from build123d import *

# Parameters (mm, degrees)
SKETCH1_W           = 29.083
SKETCH1_H           = 13.0302
BOSS_EXTRUDE1_DEPTH = 19.0754
SKETCH2_W           = 39.9542
SKETCH2_H           = 13.0302
BOSS_EXTRUDE2_DEPTH = 3.4798
SKETCH3_W           = 29.21
SKETCH3_H           = 12.954
BOSS_EXTRUDE3_DEPTH = 4.0132
SKETCH4_R           = 3.071074645
BOSS_EXTRUDE4_DEPTH = 4.572
SKETCH5_R           = 2.159
CUT_EXTRUDE1_DEPTH  = 3.4798


with BuildPart() as part:
    # Sketch1 → Boss-Extrude1 (new body)
    with BuildSketch(Plane(origin=(0, 0, 0), x_dir=(1, 0, 0), z_dir=(0, 1, 0))):
        Rectangle(SKETCH1_W, SKETCH1_H)
    extrude(amount=BOSS_EXTRUDE1_DEPTH)

    # Sketch2 → Boss-Extrude2 (add)
    with BuildSketch(Plane(origin=(0, 19.0754, 0), x_dir=(1, 0, 0), z_dir=(0, 1, 0))):
        Rectangle(SKETCH2_W, SKETCH2_H)
    extrude(amount=BOSS_EXTRUDE2_DEPTH)

    # Sketch3 → Boss-Extrude3 (add)
    with BuildSketch(Plane(origin=(0, 22.5552, 0), x_dir=(1, 0, 0), z_dir=(0, 1, 0))):
        with Locations((-0.0635, 0.0381)):
            Rectangle(SKETCH3_W, SKETCH3_H)
    extrude(amount=BOSS_EXTRUDE3_DEPTH)

    # Sketch4 → Boss-Extrude4 (add)
    with BuildSketch(Plane(origin=(0, 26.5684, 0), x_dir=(1, 0, 0), z_dir=(0, 1, 0))):
        with Locations(Location((-9.4771, 0, 0), (0, 0, 90))):
            Circle(SKETCH4_R)
    extrude(amount=BOSS_EXTRUDE4_DEPTH)

    # Sketch5 → Cut-Extrude1 (cut)
    with BuildSketch(Plane(origin=(0, 22.5552, 0), x_dir=(1, 0, 0), z_dir=(0, 1, 0))):
        with Locations((-17.9451, 0)):
            Circle(SKETCH5_R)
        with Locations((17.9451, 0)):
            Circle(SKETCH5_R)
    extrude(amount=-CUT_EXTRUDE1_DEPTH, mode=Mode.SUBTRACT)


solid = part.part
Input: part model. Units: mm. Frame: model coordinates. A direction names the side the tool comes from. Round coordinates to 2 decimals unless told otherwise and drop trailing zeros. Loops run counter-clockwise (first coordinate to the right, second up) from the corner with the lowest first, then second, coordinate; pieces in that order, holes last. Notation, with made-up numbers: M 26,-9 L 79,-9 A34 ccw 79,27 Z; hole C 84,55 d11. An arc over 180 degrees is marked long. Answer as CSV lines item,"result". Start each with the question number.
(1) Section D-D, the plane y = 28.5. Output: boundary loops of the cut face in (x, z).
(2) First-contact query: pin 1 (5 mm diameter, centred on x = -17.95, z = 0, fed in from +Y); pin 2 (6.5 mm diameter, centred on y = 9.5, z = -1, fed in from -X); pin 3 (1.2 mm diameter, centred on y = 25.5, z = 1, fed in from +X). Flat tips, straight axial feed; report the tip coordinate or a pass-through.
(3) Section B-B, the plane x = -0.5. Output: boundary loops of the cut face in (y, z), plus the area to 3 significant figures.
(4) Section C-C, the plane z = -3.75. Output: boundary loops of the cut face in (x, y).
(5) Section A-A, the plane z = 0. Output: boundary loops of the cut face in (x, y), plus the area to 3 significant figures.
(6) Draft query along Z for faces 6 (the cylindrical face through (-15.788, 20.84, 0.085)), 7 (the cylindrical face through (-12.52, 28.82, 0.4)), 8 (the flat face through (0, 25, 6.439)), 9 (the flat face through (-10, 31.14, 0)). Return one class per face: released by +Z, released by -Z, zero draft, split by the parting line, or undercut.
(7) Reachability of faces 1 (the flat face through (19.977, 21, 4)), 2 (the flat face through (-14.668, 25, 0)), 3 (the flat face through (-14.542, 9, 0)), 4 (the flat face through (14.542, 25, 0)), 5 (the flat face through (15, 19.075, 0)) from +Z, -Z, +X, -X, +Y, -Y: full face, straight path, thin tool, end or side. Return the list, or none.
(8) Line query: line 1 (X direction, y = 20, z = 0); line 2 (Y direction, x = -0.5, z = 4); line 3 (X direction, y = 19, z = 0.75). Output: solid intervals per line, ascending. Write a range as [from, to].
Values found:
1,outline,"C -9.48,0 d6.14"
2,pin 1,"stops at y = 22.56"
2,pin 2,"stops at x = -14.54"
2,pin 3,"stops at x = 14.54"
3,outline,"M 0,-6.52 L 26.57,-6.52 L 26.57,6.44 L 22.56,6.44 L 22.56,6.52 L 0,6.52 Z"
3,area,"346 mm²"
4,outline,"M -19.98,19.08 L -14.54,19.08 L -14.54,0 L 14.54,0 L 14.54,19.08 L 19.98,19.08 L 19.98,22.56 L 14.54,22.56 L 14.54,26.57 L -14.67,26.57 L -14.67,22.56 L -19.98,22.56 Z"
5,outline,"M -15.79,19.08 L -14.54,19.08 L -14.54,0 L 14.54,0 L 14.54,19.08 L 15.79,19.08 L 15.79,22.56 L 14.54,22.56 L 14.54,26.57 L -6.41,26.57 L -6.41,31.14 L -12.55,31.14 L -12.55,26.57 L -14.67,26.57 L -14.67,22.56 L -15.79,22.56 Z"
5,area,"810 mm²"
6,face 6,"undercut"
6,face 7,"split by the parting line"
6,face 8,"released by +Z"
6,face 9,"zero draft"
7,face 1,"+Z, -Z, +X, +Y, -Y"
7,face 2,"+Z, -Z, -X, +Y"
7,face 3,"+Z, -Z, -X, -Y"
7,face 4,"+Z, -Z, +X, +Y"
7,face 5,"+Z, -Z, +X, -Y"
8,line 1,"x = [-15.79, 15.79]"
8,line 2,"y = [0, 26.57]"
8,line 3,"x = [-14.54, 14.54]"
